from build123d import *

# Parameters (mm, degrees)
MODEL_R         = 1.5
MODEL_W         = 9.700000003
MODEL_H         = 1.95
MODEL_W_2       = 1.95
MODEL_H_2       = 9.700000003
MODEL_H_3       = 9.7
EXTRUDE_1_DEPTH = 3


with BuildPart() as part:
    # Model → Бобышка-Вытянуть1 (new body)
    with BuildSketch(Plane.XY):
        with BuildLine():
            Line((36, -10), (57.083920217, -10))
            ThreePointArc((57.083920217, -10), (59.02041189, -9.291287847), (60.041960108, -7.5))
            ThreePointArc((60.041960108, -7.5), (60.878679656, -5.878679656), (62.5, -5.041960108))
            ThreePointArc((62.5, -5.041960108), (64.291287847, -4.02041189), (65, -2.083920217))
            Line((65, -2.083920217), (65, 2.083920217))
            ThreePointArc((65, 2.083920217), (64.291287847, 4.02041189), (62.5, 5.041960108))
            ThreePointArc((62.5, 5.041960108), (60.878679656, 5.878679656), (60.041960108, 7.5))
            ThreePointArc((60.041960108, 7.5), (59.02041189, 9.291287847), (57.083920217, 10))
            Line((57.083920217, 10), (36, 10))
            ThreePointArc((36, 10), (31.757359313, 11.757359313), (30, 16))
            Line((30, 16), (30, 60))
            ThreePointArc((30, 60), (29.121320344, 62.121320344), (27, 63))
            Line((27, 63), (8, 63))
            ThreePointArc((8, 63), (5.878679656, 63.878679656), (5, 66))
            Line((5, 66), (5, 67))
            ThreePointArc((5, 67), (4.121320344, 69.121320344), (2, 70))
            Line((2, 70), (-2, 70))
            ThreePointArc((-2, 70), (-4.121320344, 69.121320344), (-5, 67))
            Line((-5, 67), (-5, 66))
            ThreePointArc((-5, 66), (-5.878679656, 63.878679656), (-8, 63))
            Line((-8, 63), (-27, 63))
            ThreePointArc((-27, 63), (-29.121320344, 62.121320344), (-30, 60))
            Line((-30, 60), (-30, 16))
            ThreePointArc((-30, 16), (-31.757359313, 11.757359313), (-36, 10))
            Line((-36, 10), (-57.083920217, 10))
            ThreePointArc((-57.083920217, 10), (-59.02041189, 9.291287847), (-60.041960108, 7.5))
            ThreePointArc((-60.041960108, 7.5), (-60.878679656, 5.878679656), (-62.5, 5.041960108))
            ThreePointArc((-62.5, 5.041960108), (-64.291287847, 4.02041189), (-65, 2.083920217))
            Line((-65, 2.083920217), (-65, -2.083920217))
            ThreePointArc((-65, -2.083920217), (-64.291287847, -4.02041189), (-62.5, -5.041960108))
            ThreePointArc((-62.5, -5.041960108), (-60.878679656, -5.878679656), (-60.041960108, -7.5))
            ThreePointArc((-60.041960108, -7.5), (-59.02041189, -9.291287847), (-57.083920217, -10))
            Line((-57.083920217, -10), (-36, -10))
            ThreePointArc((-36, -10), (-31.757359313, -11.757359313), (-30, -16))
            Line((-30, -16), (-30, -60))
            ThreePointArc((-30, -60), (-29.121320344, -62.121320344), (-27, -63))
            Line((-27, -63), (8, -63))
            Line((8, -63), (27, -63))
            ThreePointArc((27, -63), (29.121320344, -62.121320344), (30, -60))
            Line((30, -60), (30, -16))
            ThreePointArc((30, -16), (31.757359313, -11.757359313), (36, -10))
        make_face()
        Circle(MODEL_R, mode=Mode.SUBTRACT)
        with Locations((0, 66)):
            Circle(MODEL_R, mode=Mode.SUBTRACT)
        with Locations((61, 0)):
            Circle(MODEL_R, mode=Mode.SUBTRACT)
        with Locations((-61, 0)):
            Circle(MODEL_R, mode=Mode.SUBTRACT)
        with Locations((-29.000000002, -6)):
            Rectangle(MODEL_W, MODEL_H, mode=Mode.SUBTRACT)
        with Locations((28.999999999, -6)):
            Rectangle(MODEL_W, MODEL_H, mode=Mode.SUBTRACT)
        with Locations((49, -1e-09)):
            Rectangle(MODEL_W_2, MODEL_H_2, mode=Mode.SUBTRACT)
        with Locations((-49, 0)):
            Rectangle(MODEL_W_2, MODEL_H_3, mode=Mode.SUBTRACT)
        with Locations((-56.5, 0)):
            Rectangle(MODEL_W_2, MODEL_H_3, mode=Mode.SUBTRACT)
        with Locations((56.5, 0)):
            Rectangle(MODEL_W_2, MODEL_H_3, mode=Mode.SUBTRACT)
        with BuildLine():
            Line((-16.5, 10.5), (16.5, 10.5))
            ThreePointArc((16.5, 10.5), (20.742640687, 12.257359313), (22.5, 16.5))
            Line((22.5, 16.5), (22.5, 49.5))
            ThreePointArc((22.5, 49.5), (20.742640687, 53.742640687), (16.5, 55.5))
            Line((16.5, 55.5), (-16.5, 55.5))
            ThreePointArc((-16.5, 55.5), (-20.742640687, 53.742640687), (-22.5, 49.5))
            Line((-22.5, 49.5), (-22.5, 16.5))
            ThreePointArc((-22.5, 16.5), (-20.742640687, 12.257359313), (-16.5, 10.5))
        make_face(mode=Mode.SUBTRACT)
        with BuildLine():
            Line((-16.5, -10.5), (16.5, -10.5))
            ThreePointArc((16.5, -10.5), (20.742640687, -12.257359313), (22.5, -16.5))
            Line((22.5, -16.5), (22.5, -49.5))
            ThreePointArc((22.5, -49.5), (20.742640687, -53.742640687), (16.5, -55.5))
            Line((16.5, -55.5), (-16.5, -55.5))
            ThreePointArc((-16.5, -55.5), (-20.742640687, -53.742640687), (-22.5, -49.5))
            Line((-22.5, -49.5), (-22.5, -16.5))
            ThreePointArc((-22.5, -16.5), (-20.742640687, -12.257359313), (-16.5, -10.5))
        make_face(mode=Mode.SUBTRACT)
    extrude(amount=EXTRUDE_1_DEPTH)


solid = part.part
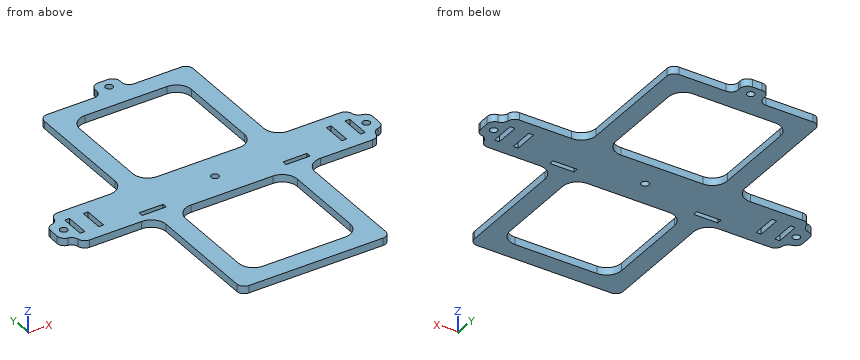
Verification items for the finished model (mm, model axes). Give positions to 0.01 mm unless a question says otherwise; leave off trailing zeros. Loops run counter-clockwise (first coordinate to the right, second up) from the corner with the lowest first, then second, coordinate; pieces in that order, holes last.
1) Sectioned sample at A-A, the plane x = 0. Enter the section's corners in (y, z), then the cut area to 3 significant figures.
2) Sectioned sample at D-D, the plane x = -21. Enter the section's corners in (y, z), then the cut area to 3 significant figures.
3) Sectioned sample at C-C, the plane y = 0. Count the separate pieces of the cut face and the enclosed holes in it, then the cut area to 3 significant figures.
4) Depth check by flat-ended pin: pin 1 Ø0.6 at (x, z) = (49, 1.5) entering from +Y; pin 2 Ø1.6 at (x, z) = (48.5, 1.5) entering from -Y; pin 3 Ø1.8 at (x, y) = (61, 0) entering from -Z; pin 4 Ø0.9 at (x, z) = (13.5, 2) entering from +Y. Enter the tip coordinate at first touch or a pass-through.
5) Sectioned sample at B-B, the plane y = -21. Enter the section's corners in (x, z).
6) Thickness scan on line 1 along Y through (x, z) = (0, 0.85); line 2 along Y through (x, z) = (-13.5, 2); line 3 along X through (y, z) = (45, 0.1). Record the ranges inside material, lowest first.
Answers:
1. outline: (-63, 0) - (-55.5, 0) - (-55.5, 3) - (-63, 3) - close; (-10.5, 0) - (-1.5, 0) - (-1.5, 3) - (-10.5, 3) - close; (1.5, 0) - (10.5, 0) - (10.5, 3) - (1.5, 3) - close; (55.5, 0) - (64.5, 0) - (64.5, 3) - (55.5, 3) - close; (67.5, 0) - (70, 0) - (70, 3) - (67.5, 3) - close
1. area: 111 mm2
2. outline: (-63, 0) - (-53.47, 0) - (-53.47, 3) - (-63, 3) - close; (-12.53, 0) - (12.53, 0) - (12.53, 3) - (-12.53, 3) - close; (53.47, 0) - (63, 0) - (63, 3) - (53.47, 3) - close
2. area: 132 mm2
3. separate pieces: 8
3. enclosed holes: 0
3. area: 340 mm2
4. pin 1: stops at y = 10
4. pin 2: stops at y = -10
4. pin 3: passes through
4. pin 4: stops at y = 63
5. outline: (-30, 0) - (-22.5, 0) - (-22.5, 3) - (-30, 3) - close; (22.5, 0) - (30, 0) - (30, 3) - (22.5, 3) - close
6. line 1: y = -63 to -55.5, -10.5 to -1.5, 1.5 to 10.5, 55.5 to 64.5, 67.5 to 70
6. line 2: y = -63 to -55.5, -10.5 to 10.5, 55.5 to 63
6. line 3: x = -30 to -22.5, 22.5 to 30
